The model under review builds one solid part; all positions refer to its coordinate system, in mm. A direction names the side the tool comes from. Coordinates: 2 decimals unless noted, no trailing zeros. Order: outer loops, then holes, each group sorted by start corner. A loop starts at its lowest first (then second) coordinate and runs counter-clockwise, first axis right, second up. Notation, with made-up numbers: M 35.5,2.5 L 94.5,2.5 A21 cw 94.5,35.5 Z; hole C -29,-14 d8. An arc over 180 degrees is marked long. Write each question's results on one line, items separated by ' | '.
from build123d import *

# Parameters (mm, degrees)
F0_R     = 29.5
F1_DEPTH = 72
F3_SIZE2 = 11.5
F3_SIZE  = 8
F4_R     = 4
F5_DEPTH = 103
F7_D     = 4
F7_DEPTH = 20
F7_TIP   = 1.2017212381


# Not quite as in the source:
# - a fillet or chamfer that OpenCascade refuses, or shapes differently, is made with other operations: its cross-section is extruded or revolved along the edge and cut away or added


with BuildPart() as f1:
    # F0 (on Top) → F1 (new body)
    with BuildSketch(Plane.XY):
        Circle(F0_R)
    extrude(amount=F1_DEPTH)

    # F2: chamfer of 3.5 x 10 on 1 edges, made by hand

    # F2_s1 → F2_t2 (revolve, cut)
    with BuildSketch(Plane.XZ):
        Polygon((29.5, 62), (26, 72), (29.5, 72), align=None)
    revolve(axis=Axis((0, 0, 72), (0, 0, 1)), mode=Mode.SUBTRACT)

    # F3
    f3_edges = [f1.edges().sort_by_distance(p)[0] for p in [
        (-29.5, 0, 0),
    ]]
    chamfer(f3_edges, length=F3_SIZE, length2=F3_SIZE2)

    # F4 (on Top) → F5 (join)
    with BuildSketch(Plane.XY):
        Circle(F4_R)
    extrude(amount=F5_DEPTH)

    # F7
    with Locations(Plane.XY.offset(72)):
        with Locations((0, 22.5), (22.5, 0), (0, -22.5), (-22.5, 0)):
            Hole(F7_D / 2, depth=F7_DEPTH)
            with Locations((0, 0, -(F7_DEPTH + F7_TIP / 2))):  # 118° drill point
                Cone(0, F7_D / 2, F7_TIP, mode=Mode.SUBTRACT)


solid = f1.part
1) The part is to be moulded in two halves that separate along X. For faces 1 (the conical face through (-4.02, -18.12, 0.39)), 2 (the flat face through (0, 0, 103)), 3 (the cylindrical face through (0.26, -20.517, 61.86)), say which applies: pulls with the +X half, pulls with the -X half, needs draft (parallel to the pull), parting line crosses it, or undercut.
Solutions:
face 1: parting line crosses it | face 2: needs draft | face 3: undercut
2) For faces 4 (the cylindrical face through (24.1, -1.2, 61.9)), 5 (the flat face through (0, 0, 0)), list the 3-axis set-ups (+Z, -Z, +X, -X, +Y, -Y) from which the entire face can be reached by the end or side of a thin tool; tool diameter is ignored.
Solutions:
face 4: +Z | face 5: -Z, +X, -X, +Y, -Y
3) Take a section at A-A on z = 67. State the section outline as (x, y) points.
Solutions:
outline: C 0,0 d55.5; hole C -22.5,0 d4; hole C 0,-22.5 d4; hole C 0,22.5 d4; hole C 22.5,0 d4
4) To check wall thickness, follow line 1 along Z through (x, y) = (-13.5, 5); line 2 along X through (y, z) = (-1, 38.5); line 3 along X through (y, z) = (0, 64). State the ranges of each line that lie inside material, in increasing order.
Solutions:
line 1: 0 to 72 | line 2: -29.48 to 29.48 | line 3: -28.8 to -24.5, -20.5 to 20.5, 24.5 to 28.8
5) For pin 1 (1 mm diameter, centred on x = 21, y = -8, fed in from -Z); pin 2 (1.5 mm diameter, centred on x = -21.5, z = 25.5, fed in from +Y); pin 3 (3.5 mm diameter, centred on x = 0, y = 22.5, fed in from -Z), all flat-tipped, find the tip position at first contact; note any pin that passes through.
Solutions:
pin 1: z = 2.76 | pin 2: y = 20.97 | pin 3: z = 1.91
6) Take a section at B-B on z = 14. State the section outline as (x, y) points, plus the area to 3 significant figures.
Solutions:
outline: C 0,0 d59 | area: 2,730 mm2
